```python
from build123d import *

# Parameters (mm, degrees)
SKETCH1_R           = 47
SKETCH1_R_2         = 45
BOSS_EXTRUDE1_DEPTH = 6
SKETCH4_R           = 2.5


with BuildPart() as part:
    # Sketch1 → Boss-Extrude1 (new body)
    with BuildSketch(Plane(origin=(0, 0, 0), x_dir=(1, 0, 0), z_dir=(0, 1, 0))):
        Circle(SKETCH1_R)
        Circle(SKETCH1_R_2, mode=Mode.SUBTRACT)
    extrude(amount=BOSS_EXTRUDE1_DEPTH)

    # Sketch4 → Cut-Revolve2 (revolve, cut)
    with BuildSketch(Plane(origin=(0, 0, 0), x_dir=(0, 0, -1), z_dir=(1, 0, 0))):
        with Locations((-48.2, 3)):
            Circle(SKETCH4_R)
    revolve(axis=Axis((0, 0, 0), (0, 1, 0)), mode=Mode.SUBTRACT)


solid = part.part
```
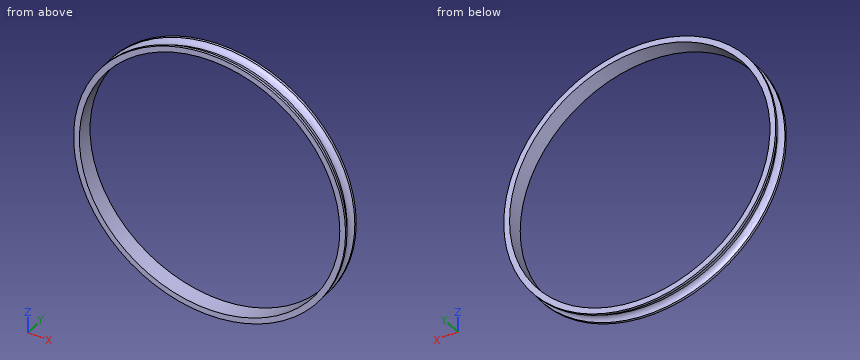
For this review, take the finished solid that the model builds, in its own axes (mm). Coordinates: 2 decimals unless noted, no trailing zeros. Order: outer loops, then holes, each group sorted by start corner. A loop starts at its lowest first (then second) coordinate and runs counter-clockwise, first axis right, second up. Notation, with made-up numbers: (6, 49.25) - (58, 49.25) arc R34 ccw to (58, 80.25) - close; hole circle Ø10 at (14.5, 64). An arc over 180 degrees is marked (long way). Answer as a JSON object with one key per item and string values. Group by question number.
1. Clearance check with flat-ended pins moving along their axes: P1, Ø2, axis at x = 15.5, y = 2, coming from the +Z side; P2, Ø1, axis at x = -2, y = 2, coming from the -Z side; P3, Ø1.5, axis at y = 1, z = 13, coming from the +X side. State where each tip first meets the part, or that it passes through.
2. We need section A-A on z = 0. State the section outline as (x, y) points.
3. We need section B-B on x = 0. State the section outline as (y, z) points.
4. For probe 1 along X at (y, z) = (0.35, -12); probe 2 along Z at (x, y) = (36.5, 3); probe 3 along Z at (x, y) = (20, 2.65), list the stretches that pass through material, from the lowest coordinate up.
Final values:
{
 "1": {"P1": "z = 44.1", "P2": "z = -46.16", "P3": "x = 45.37"},
 "2": {"outline": "(-47, 0) - (-45, 0) - (-45, 6) - (-47, 6) - (-47, 5.19) arc R2.5 cw to (-47, 0.81) - close; (45, 0) - (47, 0) - (47, 0.81) arc R2.5 cw to (47, 5.19) - (47, 6) - (45, 6) - close"},
 "3": {"outline": "(0, -47) - (0.81, -47) arc R2.5 cw to (5.19, -47) - (6, -47) - (6, -45) - (0, -45) - close; (0, 45) - (6, 45) - (6, 47) - (5.19, 47) arc R2.5 cw to (0.81, 47) - (0, 47) - close"},
 "4": {"probe 1": "-45.44 to -43.37, 43.37 to 45.44", "probe 2": "-27.5 to -26.32, 26.32 to 27.5", "probe 3": "-41.12 to -40.31, 40.31 to 41.12"}
}
